Verification items for the finished model (mm, model axes). A direction names the side the tool comes from. Round coordinates to 2 decimals unless told otherwise and drop trailing zeros. Loops run counter-clockwise (first coordinate to the right, second up) from the corner with the lowest first, then second, coordinate; pieces in that order, holes last. Notation, with made-up numbers: (-22.75, 19.5) - (30.25, 19.5) arc R11 ccw to (30.25, 27.5) - close; hole circle Ø2 at (-18, 46). An arc over 180 degrees is marked (long way). Use CSV: the item, a comma, the result in double quotes.
```python
from build123d import *

# Parameters (mm, degrees)
F_3_0_3_DIAMETER_HOLE1_D = 3
M2_5_TAPPED_HOLE1_D      = 2.05
CIRPATTERN1_COUNT        = 8
F_2_0_2_DIAMETER_HOLE1_D = 2
M2_TAPPED_HOLE1_D        = 1.6
CIRPATTERN2_COUNT        = 4
SKETCH14_R               = 3.5
CUT_EXTRUDE1_DEPTH       = 4


with BuildPart() as part:
    # Sketch1 → Revolve1 (revolve)
    with BuildSketch(Plane.XZ, mode=Mode.PRIVATE) as revolve1_sk:
        Polygon((2.75, 25), (0, 25), (0, 24.516404416), (0, 20.5), (5.5, 20.5), (5.5, 21), (14, 21), (14, 23.5), (5, 23.5), (5, 25), align=None)
    revolve(revolve1_sk.sketch.rotate(Axis((0, 0, 24.516404416), (0, 0, -1)), 180), axis=Axis((0, 0, 24.516404416), (0, 0, -1)))

    # Ø3.0 (3) Diameter Hole1 (through all)
    with Locations(Plane.XY.offset(25)):
        with Locations((0, 0)):
            Hole(F_3_0_3_DIAMETER_HOLE1_D / 2)

    # M2.5 Tapped Hole1 (through all)
    with Locations(Plane.XY.offset(23.5)):
        with Locations((0, 11)):
            m2_5_tapped_hole1 = Hole(M2_5_TAPPED_HOLE1_D / 2)

    # CirPattern1: M2.5 Tapped Hole1 ×8 about axis
    cirpattern1_axis = Axis((0, 0, 0), (0, 0, 1))
    for i in range(1, CIRPATTERN1_COUNT):
        add(m2_5_tapped_hole1.rotate(cirpattern1_axis, i * 360 / CIRPATTERN1_COUNT), mode=Mode.SUBTRACT)

    # Ø2.0 (2) Diameter Hole1 (through all)
    with Locations(Plane.XY.offset(25)):
        with Locations((0, 8), (8, 0), (0, -8), (-8, 0)):
            Hole(F_2_0_2_DIAMETER_HOLE1_D / 2)

    # M2 Tapped Hole1 (through all)
    with Locations(Plane.XY.offset(23.5)):
        with Locations((5.656854249, 5.656854249)):
            m2_tapped_hole1 = Hole(M2_TAPPED_HOLE1_D / 2)

    # CirPattern2: M2 Tapped Hole1 ×4 about axis
    cirpattern2_axis = Axis((0, 0, 0), (0, 0, 1))
    for i in range(1, CIRPATTERN2_COUNT):
        add(m2_tapped_hole1.rotate(cirpattern2_axis, i * 360 / CIRPATTERN2_COUNT), mode=Mode.SUBTRACT)

    # Sketch14 → Cut-Extrude1 (cut)
    with BuildSketch(Plane(origin=(0, 0, 20.5), x_dir=(-1, 0, 0), z_dir=(0, 0, -1))):
        Circle(SKETCH14_R)
    extrude(amount=-CUT_EXTRUDE1_DEPTH, mode=Mode.SUBTRACT)


solid = part.part
```
1) Thickness scan on probe 1 along Y at (x, z) = (0, 22.15) (3 decimals); probe 2 along Y at (x, z) = (0, 24.7); probe 3 along Y at (x, z) = (-8, 22.4). Record the ranges inside material, lowest first. Write a range as [from, to].
Returned:
probe 1,"y = [-14, -12.025], [-9.975, -9], [-7, -3.5], [3.5, 7], [9, 9.975], [12.025, 14]"
probe 2,"y = [-5, -1.5], [1.5, 5]"
probe 3,"y = [-11.49, -8.78], [-6.78, -1], [1, 6.78], [8.78, 11.49]"
2) Access from +Z, -Z, +X, -X, +Y, -Y to the whole of each face (thin tool, end or side, straight path). Record for faces 4 (the face through (0, -6, 23.5)), 5 (the face through (-3.233, -1.341, 22.472)), 6 (the face through (-8.534, -7.086, 22.232)).
Returned:
face 4,"+Z"
face 5,"-Z"
face 6,"+Z, -Z"
3) Mould release check, pull along Y, two halves, no side actions. Record for faces 1 (the face through (0.551, -11.864, 22.232)), 2 (the face through (4, 0, 20.5)), 3 (the face through (1.19, -5.37, 20.75)): +Y half, -Y half, draft (parallel to the pull), parting line (faces both ways), or undercut.
Returned:
face 1,"undercut"
face 2,"draft"
face 3,"parting line"
4) Cross-section at A-A, the plane y = -11. Record the cut outline in (x, z) (3 decimals), then the cut area to 3 significant figures.
Returned:
outline,"(-8.66, 21) - (-1.025, 21) - (-1.025, 23.5) - (-8.66, 23.5) - close; (1.025, 21) - (8.66, 21) - (8.66, 23.5) - (1.025, 23.5) - close"
area,"38.2 mm²"
5) Cross-section at B-B, the plane x = 0. Count the separate pieces of the cut face and the enclosed holes in it, then the cut area to 4 significant figures.
Returned:
separate pieces,"6"
enclosed holes,"0"
area,"40.75 mm²"
6) Cross-section at D-D, the plane y = -8. Record the cut outline in (x, z), then the cut area to 3 significant figures.
Returned:
outline,"(-11.49, 21) - (-8.78, 21) - (-8.78, 23.5) - (-11.49, 23.5) - close; (-6.78, 21) - (-1, 21) - (-1, 23.5) - (-6.78, 23.5) - close; (1, 21) - (6.78, 21) - (6.78, 23.5) - (1, 23.5) - close; (8.78, 21) - (11.49, 21) - (11.49, 23.5) - (8.78, 23.5) - close"
area,"42.4 mm²"
7) Gauge pin test, flat ends, axial feed: pin 1 Ø1.5 at (x, z) = (3.5, 22.5) entering from +Y; pin 2 Ø3.5 at (x, y) = (0, -11) entering from -Z; pin 3 Ø5.5 at (x, y) = (0, 0) entering from -Z. Record the tip position at first contact, or that the pin passes through.
Returned:
pin 1,"stops at y = 13.73"
pin 2,"stops at z = 21"
pin 3,"stops at z = 24.5"
